Source: three-view drawing plus pictorial views. Frame: mm from the lowest corner of the part. Round coordinates to 2 decimals unless told otherwise and drop trailing zeros. Loops run counter-clockwise (first coordinate to the right, second up) from the corner with the lowest first, then second, coordinate; pieces in that order, holes last. Notation, with made-up numbers: M -38.5,-8 L 18.5,-8 A17 cw 18.5,25 Z; hole C 70.25,-30 d5. An arc over 180 degrees is marked long. Return JSON: item names as keys, results as strings. Group by question number.
1) Section A-A (x = 33). Output: boundary loops of the cut face in (y, z), plus the area to 3 significant figures.
2) Section C-C (y = 2.25). Output: boundary loops of the cut face in (x, z).
3) Section B-B (z = 34.5). Output: boundary loops of the cut face in (x, y).
4) Material intervals for line 1 (Z direction, x = 57, y = 3.2); line 2 (Z direction, x = 6, y = 4.15); line 3 (Z direction, x = 91, y = 2.1), sorted ascending. Write a range as from..to.
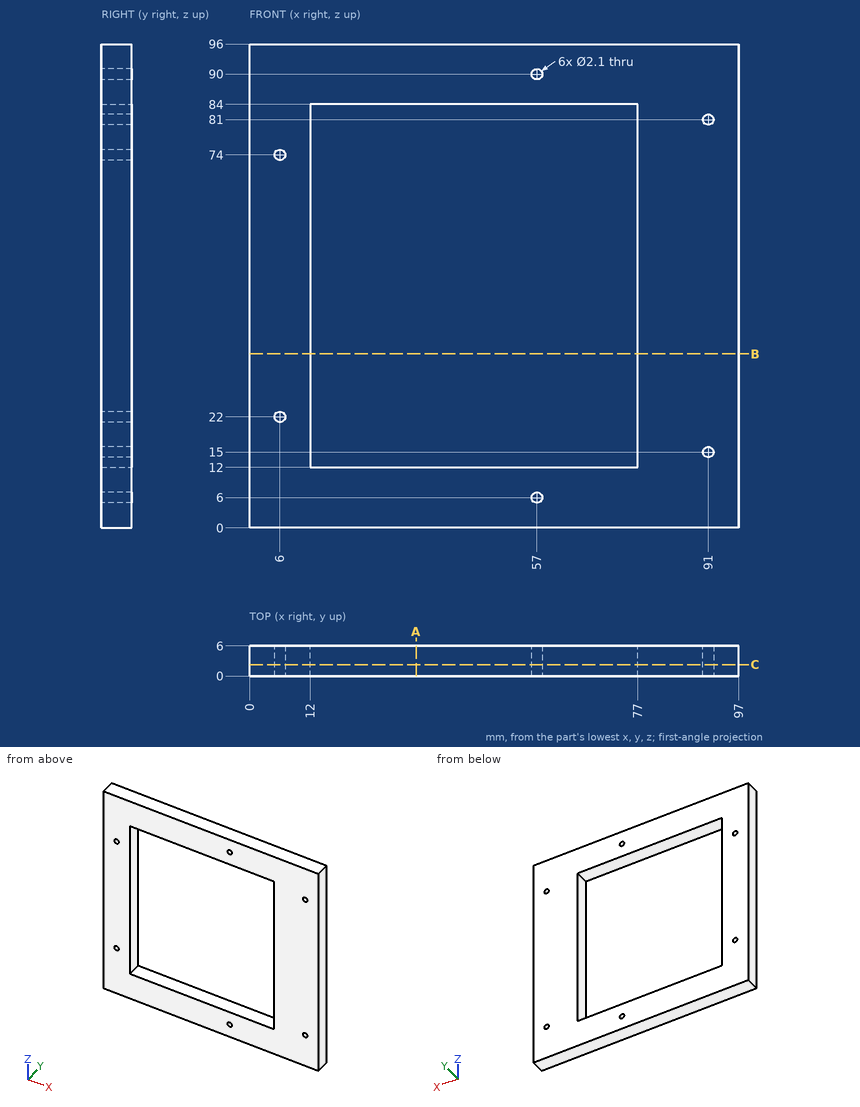
Returned:
{
 "1": {"outline": "M 0,0 L 6,0 L 6,12 L 0,12 Z; M 0,84 L 6,84 L 6,96 L 0,96 Z", "area": "144 mm^2"},
 "2": {"outline": "M 0,0 L 97,0 L 97,96 L 0,96 Z; hole C 6,22 d2.1; hole C 6,74 d2.1; hole M 12,12 L 77,12 L 77,84 L 12,84 Z; hole C 57,6 d2.1; hole C 57,90 d2.1; hole C 91,15 d2.1; hole C 91,81 d2.1"},
 "3": {"outline": "M 0,0 L 12,0 L 12,6 L 0,6 Z; M 77,0 L 97,0 L 97,6 L 77,6 Z"},
 "4": {"line 1": "z = 0..4.95, 7.05..12, 84..88.95, 91.05..96", "line 2": "z = 0..20.95, 23.05..72.95, 75.05..96", "line 3": "z = 0..13.95, 16.05..79.95, 82.05..96"}
}
